from build123d import *

# Parameters (mm, degrees)
BOSS_EXTRUDE1_DEPTH     = 1.2
FILLET1_R               = 3.5
FILLET2_R               = 5
FILLET3_R               = 2
SKETCH3_R               = 1.2
CUT_EXTRUDE1_DEPTH      = 47.412929356
MIRROR2_COPY_1_SKETCH_R = 1.2
MIRROR2_COPY_1_DEPTH    = 47.412929356


with BuildPart() as part:
    # Sketch2 → Boss-Extrude1 (new, symmetric)
    with BuildSketch(Plane(origin=(0, 0, 0), x_dir=(1, 0, 0), z_dir=(0, 1, 0))):
        Polygon((-34.5, -17.5), (-34.5, 17.5), (-19.164918189, 17.456295518), (-23.435988128, 24.29000742), (-11.564011872, 31.70999258), (-7.623299146, 25.404852218), (7.623299146, 25.404852218), (11.564011872, 31.70999258), (23.435988128, 24.29000742), (19.164918189, 17.456295518), (34.5, 17.5), (34.5, -17.5), (19.164918189, -17.456295518), (23.435988128, -24.29000742), (11.564011872, -31.70999258), (7.623299146, -25.404852218), (-7.623299146, -25.404852218), (-11.564011872, -31.70999258), (-23.435988128, -24.29000742), (-19.164918189, -17.456295518), align=None)
    extrude(amount=BOSS_EXTRUDE1_DEPTH, both=True)

    # Fillet1
    fillet1_edges = [part.edges().sort_by_distance(p)[0] for p in [
        (-19.164918189, 0, -17.456295518),
        (19.164918189, 0, -17.456295518),
        (19.164918189, 0, 17.456295518),
        (-19.164918189, 0, 17.456295518),
    ]]
    fillet(fillet1_edges, radius=FILLET1_R)

    # Fillet2
    fillet2_edges = [part.edges().sort_by_distance(p)[0] for p in [
        (-7.623299146, 0, -25.404852218),
        (7.623299146, 0, -25.404852218),
        (7.623299146, 0, 25.404852218),
        (-7.623299146, 0, 25.404852218),
    ]]
    fillet(fillet2_edges, radius=FILLET2_R)

    # Fillet3
    fillet3_edges = [part.edges().sort_by_distance(p)[0] for p in [
        (34.5, 0, -17.5),
        (23.435988128, 0, -24.29000742),
        (34.5, 0, 17.5),
        (23.435988128, 0, 24.29000742),
        (11.564011872, 0, 31.70999258),
        (11.564011872, 0, -31.70999258),
        (-11.564011872, 0, -31.70999258),
        (-23.435988128, 0, -24.29000742),
        (-34.5, 0, -17.5),
        (-34.5, 0, 17.5),
        (-11.564011872, 0, 31.70999258),
        (-23.435988128, 0, 24.29000742),
    ]]
    fillet(fillet3_edges, radius=FILLET3_R)

    # Sketch3 → Cut-Extrude1 (cut, through all)
    with BuildSketch(Plane(origin=(0, 1.2, 0), x_dir=(1, 0, 0), z_dir=(0, 1, 0))):
        with Locations(Location((-16.127132138, 25.803411421, 0), (0, 0, 270))):
            Circle(SKETCH3_R)
        with Locations(Location((-11.330641731, 26.147910732, 0), (0, 0, 270))):
            Circle(SKETCH3_R)
        with Locations(Location((-18.538627315, 21.642919742, 0), (0, 0, 270))):
            Circle(SKETCH3_R)
    cut_extrude1 = extrude(amount=-CUT_EXTRUDE1_DEPTH, mode=Mode.SUBTRACT)

    # Mirror1: Cut-Extrude1 across plane
    add(cut_extrude1.mirror(Plane(origin=(0, 0, 0), x_dir=(0, 0, 1), z_dir=(1, 0, 0))), mode=Mode.SUBTRACT)

    # Mirror2: Cut-Extrude1 across plane
    add(cut_extrude1.mirror(Plane.XY), mode=Mode.SUBTRACT)

    # Mirror2 copy 1 sketch → Mirror2 copy 1 (cut, through all)
    with BuildSketch(Plane(origin=(0, 1.2, 0), x_dir=(-1, 0, 0), z_dir=(0, 1, 0))):
        with Locations(Location((-16.127132138, 25.803411421, 0), (0, 0, 270))):
            Circle(MIRROR2_COPY_1_SKETCH_R)
        with Locations(Location((-11.330641731, 26.147910732, 0), (0, 0, 270))):
            Circle(MIRROR2_COPY_1_SKETCH_R)
        with Locations(Location((-18.538627315, 21.642919742, 0), (0, 0, 270))):
            Circle(MIRROR2_COPY_1_SKETCH_R)
    extrude(amount=-MIRROR2_COPY_1_DEPTH, mode=Mode.SUBTRACT)


solid = part.part
Verification items for the finished model (mm, model axes). A direction names the side the tool comes from. Give positions to 0.01 mm unless a question says otherwise; leave off trailing zeros. Order: outer loops, then holes, each group sorted by start corner. A loop starts at its lowest first (then second) coordinate and runs counter-clockwise, first axis right, second up. Notation, with made-up numbers: (33, 65) -> (61, 65) arc R15 ccw to (61, 74) -> close; hole circle Ø10 at (44.5, 3). An arc over 180 degrees is marked (long way). Answer as CSV lines item,"result".
Q1. Access from +Z, -Z, +X, -X, +Y, -Y to the whole of each face (thin tool, end or side, straight path). Record for faces 1 (the cylindrical face through (-19.269, 0.017, 22.595)), 2 (the cylindrical face through (-7.31, -0.02, -26.05)), 3 (the flat face through (0, 0, 25.405)).
Solutions:
face 1,"+Y, -Y"
face 2,"-Z, +Y, -Y"
face 3,"+Z, +Y, -Y"
Q2. Scan lines: probe 1 along Z at (x, y) = (19, -0.85); probe 2 along Z at (x, y) = (-26.5, 0.3); probe 3 along Z at (x, y) = (3, 0.7). Record each from-to range of solid material in increasing order.
Solutions:
probe 1,"z = -27.06 to -22.75, -20.54 to 20.54, 22.75 to 27.06"
probe 2,"z = -17.48 to 17.48"
probe 3,"z = -25.4 to 25.4"
Q3. Release check for a two-part mould opening along Z. For faces 4 (the cylindrical face through (7.24, -0.02, -26.01)), 5 (the cylindrical face through (-17.3, 0.02, -26.06)), 6 (the flat face through (34.5, 0, 0)), 7 (the cylindrical face through (11.772, -0.017, 30.908)) record: +Z half, -Z half, draft (parallel to the pull), parting line (faces both ways), or undercut.
Solutions:
face 4,"-Z half"
face 5,"undercut"
face 6,"draft"
face 7,"+Z half"
Q4. Sectioned sample at B-B on y = 0.65. Count the separate pieces of the cut face and the enclosed holes in it, plus the area to 3 significant figures.
Solutions:
separate pieces,"1"
enclosed holes,"12"
area,"3,250 mm²"
Q5. Sectioned sample at A-A on x = 27. Record the cut outline in (y, z).
Solutions:
outline,"(-1.2, -17.48) -> (1.2, -17.48) -> (1.2, 17.48) -> (-1.2, 17.48) -> close"
Q6. Sectioned sample at C-C on x = 2. Record the cut outline in (y, z), plus the area to 3 significant figures.
Solutions:
outline,"(-1.2, -25.4) -> (1.2, -25.4) -> (1.2, 25.4) -> (-1.2, 25.4) -> close"
area,"122 mm²"
